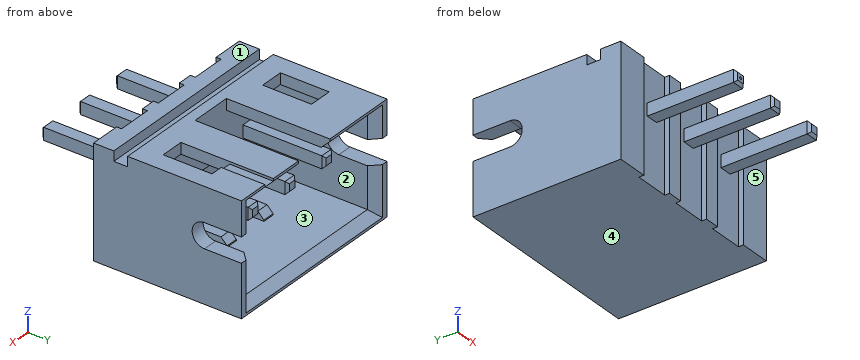
from build123d import *

# Parameters (mm, degrees)
BODY1_W                            = 7.9
BODY1_H                            = 4.5
EXTRUDE_1_DEPTH                    = 6
SKETCH_2_W                         = 6.7
SKETCH_2_H                         = 3.6
CUT_EXTRUDE_1_DEPTH                = 4.2
SKETCH_3_W                         = 7.9
SKETCH_3_H                         = 0.56
CUT_EXTRUDE_2_DEPTH                = 0.4
CHAMFER_1_SIZE                     = 0.35
CUT_EXTRUDE_3_REACH                = 12.893
SKETCH_4_W                         = 0.96
SKETCH_4_H                         = 1.98
SKETCH_5_W                         = 1.4
SKETCH_5_H                         = 0.2
CUT_EXTRUDE_4_DEPTH                = 11.893117093
SKETCH_7_W                         = 0.46
SKETCH_7_H                         = 1.77
CUT_EXTRUDE_5_DEPTH                = 0.1
CUT_EXTRUDE_6_REACH                = 12.893
SKETCH_8_W                         = 1.7
SKETCH_8_H                         = 4.2
CUT_EXTRUDE_7_REACH                = 12.893
SKETCH_15_W                        = 6.7
SKETCH_15_H                        = 1.95
CUT_EXTRUDE_9_DEPTH                = 0.65
CHAMFER_7_SIZE                     = 0.65
SKETCH_10_W                        = 0.5
SKETCH_10_H                        = 2.25
EXTRUDE_2_DEPTH                    = 0.3
CHAMFER_2_SIZE                     = 0.25
PATTERN_LINEAR_3_COUNT             = 2
PATTERN_LINEAR_3_PITCH             = 2
CHAMFER_2_OF_PATTERN_LINEAR_3_SIZE = 0.25
EXTRUDE_START                      = -4.9
SKETCH_12_W                        = 0.5
SKETCH_12_H                        = 0.5
EXTRUDE_4_DEPTH                    = 8.5
CHAMFER_3_SIZE                     = 0.1
CHAMFER_4_SIZE                     = 0.1
PATTERN_LINEAR_2_COUNT             = 3
PATTERN_LINEAR_2_PITCH             = 2
CHAMFER_3_OF_PATTERN_LINEAR_2_SIZE = 0.1
CHAMFER_4_OF_PATTERN_LINEAR_2_SIZE = 0.1
SKETCH_16_R                        = 0.05
CUT_EXTRUDE_10_DEPTH               = 3.4


with BuildPart() as part:
    # Body1 → Бобышка-Вытянуть1 (new body)
    with BuildSketch(Plane(origin=(0, 0, 0), x_dir=(1, 0, 0), z_dir=(0, 1, 0))):
        with Locations((3.95, -2.25)):
            Rectangle(BODY1_W, BODY1_H)
    extrude(amount=EXTRUDE_1_DEPTH)

    # Эскиз2 → Вырез-Вытянуть1 (cut)
    with BuildSketch(Plane(origin=(0, 6, 0), x_dir=(1, 0, 0), z_dir=(0, 1, 0))):
        with Locations((3.95, -2.25)):
            Rectangle(SKETCH_2_W, SKETCH_2_H)
    extrude(amount=-CUT_EXTRUDE_1_DEPTH, mode=Mode.SUBTRACT)

    # Эскиз3 → Вырез-Вытянуть2 (cut)
    with BuildSketch(Plane.XY.offset(4.5)):
        with Locations((3.95, 1.1)):
            Rectangle(SKETCH_3_W, SKETCH_3_H)
    extrude(amount=-CUT_EXTRUDE_2_DEPTH, mode=Mode.SUBTRACT)

    # Фаска1
    chamfer_1_edges = [part.edges().sort_by_distance(p)[0] for p in [
        (3.95, 6, 4.05),
        (7.3, 6, 2.25),
        (3.95, 6, 0.45),
        (0.6, 6, 2.25),
    ]]
    chamfer(chamfer_1_edges, length=CHAMFER_1_SIZE)

    # Эскиз4 → Вырез-Вытянуть3 (cut, up to next)
    with BuildSketch(Plane.XY.offset(4.5), mode=Mode.PRIVATE) as cut_extrude_3_sk1:
        with Locations((1.25, 3.24)):
            Rectangle(SKETCH_4_W, SKETCH_4_H)
    cut_extrude_3_tool1 = extrude(cut_extrude_3_sk1.sketch, amount=-CUT_EXTRUDE_3_REACH, mode=Mode.PRIVATE) & part.part
    # Эскиз4 → Вырез-Вытянуть3 (cut, up to next)
    with BuildSketch(Plane.XY.offset(4.5), mode=Mode.PRIVATE) as cut_extrude_3_sk2:
        with Locations((6.65, 3.24)):
            Rectangle(SKETCH_4_W, SKETCH_4_H)
    cut_extrude_3_tool2 = extrude(cut_extrude_3_sk2.sketch, amount=-CUT_EXTRUDE_3_REACH, mode=Mode.PRIVATE) & part.part
    add(cut_extrude_3_tool1.solids().sort_by_distance((1.25, 3.24, 4.5))[0], mode=Mode.SUBTRACT)
    add(cut_extrude_3_tool2.solids().sort_by_distance((6.65, 3.24, 4.5))[0], mode=Mode.SUBTRACT)

    # Эскиз5 → Вырез-Вытянуть4 (cut, through all)
    with BuildSketch(Plane.XY.offset(4.5)):
        with Locations((1.95, 0.1)):
            Rectangle(SKETCH_5_W, SKETCH_5_H)
    cut_extrude_4 = extrude(amount=-CUT_EXTRUDE_4_DEPTH, mode=Mode.SUBTRACT)

    # Эскиз7 → Вырез-Вытянуть5 (cut)
    with BuildSketch(Plane.XY.offset(4.5)):
        with Locations((6.4, 5.115)):
            Rectangle(SKETCH_7_W, SKETCH_7_H)
    extrude(amount=-CUT_EXTRUDE_5_DEPTH, mode=Mode.SUBTRACT)

    # Эскиз8 → Вырез-Вытянуть6 (cut, up to next)
    with BuildSketch(Plane.XY.offset(4.5), mode=Mode.PRIVATE) as cut_extrude_6_sk1:
        with Locations((3.95, 3.9)):
            Rectangle(SKETCH_8_W, SKETCH_8_H)
    cut_extrude_6_tool1 = extrude(cut_extrude_6_sk1.sketch, amount=-CUT_EXTRUDE_6_REACH, mode=Mode.PRIVATE) & part.part
    add(cut_extrude_6_tool1.solids().sort_by_distance((3.95, 3.9, 4.5))[0], mode=Mode.SUBTRACT)

    # Эскиз9 → Вырез-Вытянуть7 (cut, up to next)
    with BuildSketch(Plane.ZY, mode=Mode.PRIVATE) as cut_extrude_7_sk1:
        with BuildLine():
            Line((2.12, 6), (3.12, 6))
            Line((3.12, 6), (3.12, 4.5))
            ThreePointArc((3.12, 4.5), (2.62, 4), (2.12, 4.5))
            Line((2.12, 4.5), (2.12, 6))
        make_face()
    cut_extrude_7_tool1 = extrude(cut_extrude_7_sk1.sketch, amount=-CUT_EXTRUDE_7_REACH, mode=Mode.PRIVATE) & part.part
    cut_extrude_7 = cut_extrude_7_tool1.solids().sort_by_distance((0, 5.05036, 2.62))[0]
    add(cut_extrude_7, mode=Mode.SUBTRACT)

    # Зеркальное отражение1: Вырез-Вытянуть7 across plane
    add(cut_extrude_7.mirror(Plane(origin=(3.95, 0, 0), x_dir=(0, 0, 1), z_dir=(1, 0, 0))), mode=Mode.SUBTRACT)

    # Эскиз15 → Вырез-Вытянуть9 (cut)
    with BuildSketch(Plane(origin=(0, 1.8, 0), x_dir=(1, 0, 0), z_dir=(0, 1, 0))):
        with Locations((3.95, -1.425)):
            Rectangle(SKETCH_15_W, SKETCH_15_H)
    extrude(amount=-CUT_EXTRUDE_9_DEPTH, mode=Mode.SUBTRACT)

    # Фаска7
    chamfer_7_edges = [part.edges().sort_by_distance(p)[0] for p in [
        (3.95, 1.15, 2.4),
    ]]
    chamfer(chamfer_7_edges, length=CHAMFER_7_SIZE - 0.0001)  # a hair under: the kernel refuses the full size

    # Эскиз10 → Бобышка-Вытянуть2 (add)
    with BuildSketch(Plane.XY.offset(0.45)):
        with Locations((2.95, 2.275)):
            Rectangle(SKETCH_10_W, SKETCH_10_H)
    extrude_2 = extrude(amount=EXTRUDE_2_DEPTH)

    # Фаска2
    chamfer_2_edges = [part.edges().sort_by_distance(p)[0] for p in [
        (2.95, 3.4, 0.75),
    ]]
    chamfer(chamfer_2_edges, length=CHAMFER_2_SIZE)

    # Линейный массив3: Бобышка-Вытянуть2 ×2
    with Locations(*[(i * PATTERN_LINEAR_3_PITCH, 0, 0) for i in range(1, PATTERN_LINEAR_3_COUNT)]):
        add(extrude_2)

    # Фаска2 of Линейный массив3
    chamfer_2_of_pattern_linear_3_edges = [part.edges().sort_by_distance(p)[0] for p in [
        (4.95, 3.4, 0.75),
    ]]
    chamfer(chamfer_2_of_pattern_linear_3_edges, length=CHAMFER_2_OF_PATTERN_LINEAR_3_SIZE)

    # Эскиз12 → Бобышка-Вытянуть4 (add)
    with BuildSketch(Plane.XZ.offset(-0.2).offset(EXTRUDE_START)):
        with Locations((1.95, 2.8)):
            Rectangle(SKETCH_12_W, SKETCH_12_H)
    extrude_4 = extrude(amount=EXTRUDE_4_DEPTH)

    # Фаска3
    chamfer_3_edges = [part.edges().sort_by_distance(p)[0] for p in [
        (1.7, -3.4, 2.8),
        (1.95, -3.4, 2.55),
        (2.2, -3.4, 2.8),
        (1.95, -3.4, 3.05),
    ]]
    chamfer(chamfer_3_edges, length=CHAMFER_3_SIZE)

    # Фаска4
    chamfer_4_edges = [part.edges().sort_by_distance(p)[0] for p in [
        (1.7, 5.1, 2.8),
        (1.95, 5.1, 2.55),
        (2.2, 5.1, 2.8),
        (1.95, 5.1, 3.05),
    ]]
    chamfer(chamfer_4_edges, length=CHAMFER_4_SIZE)

    # Линейный массив2: Вырез-Вытянуть4, Бобышка-Вытянуть4 ×3
    with Locations(*[(i * PATTERN_LINEAR_2_PITCH, 0, 0) for i in range(1, PATTERN_LINEAR_2_COUNT)]):
        add(cut_extrude_4, mode=Mode.SUBTRACT)
        add(extrude_4)

    # Фаска3 of Линейный массив2
    chamfer_3_of_pattern_linear_2_edges = [part.edges().sort_by_distance(p)[0] for p in [
        (3.7, -3.4, 2.8),
        (3.95, -3.4, 2.55),
        (4.2, -3.4, 2.8),
        (3.95, -3.4, 3.05),
        (5.7, -3.4, 2.8),
        (5.95, -3.4, 2.55),
        (6.2, -3.4, 2.8),
        (5.95, -3.4, 3.05),
    ]]
    chamfer(chamfer_3_of_pattern_linear_2_edges, length=CHAMFER_3_OF_PATTERN_LINEAR_2_SIZE)

    # Фаска4 of Линейный массив2
    chamfer_4_of_pattern_linear_2_edges = [part.edges().sort_by_distance(p)[0] for p in [
        (3.7, 5.1, 2.8),
        (3.95, 5.1, 2.55),
        (4.2, 5.1, 2.8),
        (3.95, 5.1, 3.05),
        (5.7, 5.1, 2.8),
        (5.95, 5.1, 2.55),
        (6.2, 5.1, 2.8),
        (5.95, 5.1, 3.05),
    ]]
    chamfer(chamfer_4_of_pattern_linear_2_edges, length=CHAMFER_4_OF_PATTERN_LINEAR_2_SIZE)

    # Эскиз16 → Вырез-Вытянуть10 (cut)
    with BuildSketch(Plane.XZ):
        with Locations((1.95, 2.8)):
            Circle(SKETCH_16_R)
    extrude(amount=CUT_EXTRUDE_10_DEPTH, mode=Mode.SUBTRACT)


solid = part.part
Geometry: final body of the model. Coordinates: model frame, mm. Face numbers are marked on the shaded views. A direction names the side the tool comes from. Give positions to 0.01 mm unless a question says otherwise; leave off trailing zeros. Write each loop counter-clockwise with the first axis right and the second up, starting at its lowest first coordinate (ties: lowest second). Pieces come first, ordered by that corner, then holes. Notation, with made-up numbers: (6, 8) -> (26, 8) arc R23 cw to (26, 39) -> close; hole circle Ø10 at (-10, 20.25). An arc over 180 degrees is marked (long way). Answer in a Markdown table with one row per item.
(1) Set-up query: the marked faces 1 and 2. Return all of +Z, -Z, +X, -X, +Y, -Y with unobstructed straight access to the full face (end or side cutting, diameter ignored); none if empty.
Answers below:
| item | result |
|---|---|
| face 1 | +Z, +X, -X, +Y, -Y |
| face 2 | +Y |
(2) Ray query, line 1 along Z through (x, y) = (6.75, 5); line 2 along X through (y, z) = (3.75, 3.8); line 3 along X through (y, z) = (5, 4.15). Return the intervals inside material, ascending. Write a range as [from, to].
Answers below:
| item | result |
|---|---|
| line 1 | [0, 0.45], [4.05, 4.5] |
| line 2 | [0, 0.6], [7.3, 7.9] |
| line 3 | [0, 3.1], [4.8, 7.9] |
(3) Section query D-D on y = 1.5. Return loops of the section in (x, z).
Answers below:
| item | result |
|---|---|
| outline | (0, 0) -> (7.9, 0) -> (7.9, 4.5) -> (0, 4.5) -> close; hole (0.6, 0.45) -> (2.7, 0.45) -> (2.7, 0.75) -> (3.2, 0.75) -> (3.2, 0.45) -> (4.7, 0.45) -> (4.7, 0.75) -> (5.2, 0.75) -> (5.2, 0.45) -> (7.3, 0.45) -> (7.3, 2.1) -> (0.6, 2.1) -> close |
(4) Section query C-C on z = 3.85. Return loops of the section in (x, y), then the cut area to 3 significant figures.
Answers below:
| item | result |
|---|---|
| outline | (0, 0) -> (1.25, 0) -> (1.25, 0.2) -> (2.65, 0.2) -> (2.65, 0) -> (3.25, 0) -> (3.25, 0.2) -> (4.65, 0.2) -> (4.65, 0) -> (5.25, 0) -> (5.25, 0.2) -> (6.65, 0.2) -> (6.65, 0) -> (7.9, 0) -> (7.9, 6) -> (7.65, 6) -> (7.3, 5.65) -> (7.3, 1.8) -> (0.6, 1.8) -> (0.6, 5.65) -> (0.25, 6) -> (0, 6) -> close |
| area | 18.3 mm^2 |
(5) Section query A-A on y = 5.25. Return loops of the section in (x, z), then the cut area to 3 significant figures.
Answers below:
| item | result |
|---|---|
| outline | (0, 0) -> (7.9, 0) -> (7.9, 2.12) -> (7.3, 2.12) -> (7.3, 0.45) -> (0.6, 0.45) -> (0.6, 2.12) -> (0, 2.12) -> close; (0, 3.12) -> (0.6, 3.12) -> (0.6, 4.05) -> (3.1, 4.05) -> (3.1, 4.5) -> (0, 4.5) -> close; (4.8, 4.05) -> (7.3, 4.05) -> (7.3, 3.12) -> (7.9, 3.12) -> (7.9, 4.5) -> (6.63, 4.5) -> (6.63, 4.4) -> (6.17, 4.4) -> (6.17, 4.5) -> (4.8, 4.5) -> close |
| area | 9.42 mm^2 |
(6) Pin query (flat end, axial travel): pin 1 (1.5 mm diameter, centred on y = -1, z = 2, fed in from -X). Return the tip coordinate at first contact, or that it passes through.
Answers below:
| item | result |
|---|---|
| pin 1 | x = 1.7 |
(7) Draft query along Z for the marked faces 3, 4 and 5. Return one class per face: +Z half, -Z half, draft (parallel to the pull), parting line (faces both ways), or undercut.
Answers below:
| item | result |
|---|---|
| face 3 | undercut |
| face 4 | -Z half |
| face 5 | draft |
